Could you check a few things on this model? Use its own coordinates, in mm. A direction names the side the tool comes from. Round coordinates to 2 decimals unless told otherwise and drop trailing zeros. Loops run counter-clockwise (first coordinate to the right, second up) from the corner with the lowest first, then second, coordinate; pieces in that order, holes last. Notation, with made-up numbers: M 76,13 L 119,13 A16 ccw 119,25 Z; hole C 56.5,65.25 d6. An arc over 180 degrees is marked long. Return JSON: item names as keys, results as strings. Group by question number.
```python
from build123d import *

# Parameters (mm, degrees)
SKETCH1_W           = 25
SKETCH1_H           = 18
SKETCH1_R           = 3.5
BOSS_EXTRUDE1_DEPTH = 25
SKETCH2_W           = 20
SKETCH2_H           = 18
SKETCH2_R           = 3.96875
BOSS_EXTRUDE2_DEPTH = 4
FILLET2_R           = 3
FILLET4_R           = 3
SKETCH3_R           = 4.65
CUT_EXTRUDE1_DEPTH  = 22
SKETCH5_W           = 19
SKETCH5_H           = 12
CUT_EXTRUDE2_DEPTH  = 22
CHAMFER1_SIZE       = 1.25
CHAMFER1_SIZE2      = 4.665063509
CHAMFER2_SIZE       = 4.5
CHAMFER2_SIZE2      = 7.794228634
FILLET5_R           = 5.54
SKETCH7_W           = 3
SKETCH7_H           = 3
CUT_EXTRUDE3_DEPTH  = 6


with BuildPart() as part:
    # Sketch1 → Boss-Extrude1 (new body)
    with BuildSketch(Plane.XY):
        with Locations((12.5, 9)):
            Rectangle(SKETCH1_W, SKETCH1_H)
        with Locations((12.5, 9)):
            Circle(SKETCH1_R, mode=Mode.SUBTRACT)
    extrude(amount=BOSS_EXTRUDE1_DEPTH)

    # Sketch2 → Boss-Extrude2 (add)
    # profile 1 of 2: a face of its own
    with BuildSketch(Plane(origin=(0, 0, 0), x_dir=(-1, 0, 0), z_dir=(0, 0, -1))):
        with Locations((10, 9)):
            Rectangle(SKETCH2_W, SKETCH2_H)
        with Locations((10, 9)):
            Circle(SKETCH2_R, mode=Mode.SUBTRACT)
    # profile 2 of 2: a face of its own
    with BuildSketch(Plane(origin=(0, 0, 0), x_dir=(-1, 0, 0), z_dir=(0, 0, -1))):
        with Locations((-35, 9)):
            Rectangle(SKETCH2_W, SKETCH2_H)
        with Locations((-35, 9)):
            Circle(SKETCH2_R, mode=Mode.SUBTRACT)
    extrude(amount=-BOSS_EXTRUDE2_DEPTH)

    # Fillet2
    fillet2_edges = [part.edges().sort_by_distance(p)[0] for p in [
        (0, 9, 4),
        (-20, 0, 2),
        (-20, 18, 2),
        (45, 0, 2),
        (45, 18, 2),
        (25, 9, 4),
    ]]
    fillet(fillet2_edges, radius=FILLET2_R)

    # Fillet4
    fillet4_edges = [part.edges().sort_by_distance(p)[0] for p in [
        (12.5, 0, 25),
        (12.5, 18, 25),
        (0, 9, 25),
        (25, 9, 25),
    ]]
    fillet(fillet4_edges, radius=FILLET4_R)

    # Sketch3 → Cut-Extrude1 (cut)
    with BuildSketch(Plane(origin=(0, 0, 0), x_dir=(-1, 0, 0), z_dir=(0, 0, -1))):
        with Locations((-12.5, 9)):
            Circle(SKETCH3_R)
    extrude(amount=-CUT_EXTRUDE1_DEPTH, mode=Mode.SUBTRACT)

    # Sketch5 → Cut-Extrude2 (cut)
    with BuildSketch(Plane(origin=(0, 0, 0), x_dir=(-1, 0, 0), z_dir=(0, 0, -1))):
        with Locations((-12.5, 9)):
            Rectangle(SKETCH5_W, SKETCH5_H)
    extrude(amount=-CUT_EXTRUDE2_DEPTH, mode=Mode.SUBTRACT)

    # Chamfer1
    chamfer1_edges = [part.edges().sort_by_distance(p)[0] for p in [
        (12.5, 3, 22),
        (12.5, 15, 22),
    ]]
    chamfer1_side = [part.faces().sort_by_distance(p)[0] for p in [
        (12.5, 3.224722051, 22),
    ]]
    chamfer(chamfer1_edges, length=CHAMFER1_SIZE, length2=CHAMFER1_SIZE2, reference=chamfer1_side[0])

    # Chamfer2
    chamfer2_edges = [part.edges().sort_by_distance(p)[0] for p in [
        (22, 9, 22),
        (3, 9, 22),
    ]]
    chamfer2_side = [part.faces().sort_by_distance(p)[0] for p in [
        (21.787573542, 9, 22),
    ]]
    chamfer(chamfer2_edges, length=CHAMFER2_SIZE, length2=CHAMFER2_SIZE2, reference=chamfer2_side[0])

    # Fillet5
    # the kernel refuses this fillet: 5.54 mm, written as the material it adds along each edge
    with BuildSketch(Plane(origin=(13.422596023, 6.99868638, 32.258237225), x_dir=(-0.11302231218972587, 0.9741169476962979, -0.19576038710151827), z_dir=(-0.48705847384814693, -0.22604462437945333, -0.8436100229619524))) as fillet5_piece_1_section:
        with BuildLine():
            CenterArc((FILLET5_R * 0.877973148149, FILLET5_R), FILLET5_R, 187.435472226, 82.564527774)
            Line((-FILLET5_R * 0.113618085915, FILLET5_R * 0.870590477449), (0, 0))
            Line((0, 0), (FILLET5_R * 0.877973148149, 0))
        make_face()
    fillet5_piece_1 = extrude(amount=29.849737763, mode=Mode.PRIVATE)
    fillet5_piece_1 = split(fillet5_piece_1, bisect_by=Plane(origin=(6.414237593, 4.456810382, 22), z_dir=(0, 0, -1)), keep=Keep.TOP, mode=Mode.PRIVATE)
    fillet5_piece_1 = split(fillet5_piece_1, bisect_by=Plane(origin=(6.414237593, 0, 18.189685112), z_dir=(0, 1, 0)), keep=Keep.TOP, mode=Mode.PRIVATE)
    fillet5_piece_1 = split(fillet5_piece_1, bisect_by=Plane(origin=(0, 4.456810382, 18.189685112), z_dir=(1, 0, 0)), keep=Keep.TOP, mode=Mode.PRIVATE)
    add(fillet5_piece_1)
    with BuildSketch(Plane(origin=(11.577403977, 6.99868638, 32.258237225), x_dir=(-0.8733693623277119, -0.12606000911046675, -0.4704623588028643), z_dir=(0.48705847384814693, -0.2260446243794534, -0.8436100229619524))) as fillet5_piece_2_section:
        with BuildLine():
            CenterArc((FILLET5_R * 0.877973148149, FILLET5_R), FILLET5_R, 187.435472226, 82.564527774)
            Line((-FILLET5_R * 0.113618085915, FILLET5_R * 0.870590477449), (0, 0))
            Line((0, 0), (FILLET5_R * 0.877973148149, 0))
        make_face()
    fillet5_piece_2 = extrude(amount=29.849737763, mode=Mode.PRIVATE)
    fillet5_piece_2 = split(fillet5_piece_2, bisect_by=Plane(origin=(18.585762403, 4.456810384, 22), z_dir=(0, 0, -1)), keep=Keep.TOP, mode=Mode.PRIVATE)
    fillet5_piece_2 = split(fillet5_piece_2, bisect_by=Plane(origin=(18.585762403, 0, 18.189685124), z_dir=(0, 1, 0)), keep=Keep.TOP, mode=Mode.PRIVATE)
    fillet5_piece_2 = split(fillet5_piece_2, bisect_by=Plane(origin=(25, 4.456810384, 18.189685124), z_dir=(-1, 0, 0)), keep=Keep.TOP, mode=Mode.PRIVATE)
    add(fillet5_piece_2)
    with BuildSketch(Plane(origin=(11.577403977, 11.00131362, 32.258237225), x_dir=(0.11302231218972622, -0.9741169476962979, -0.19576038710151802), z_dir=(0.48705847384814693, 0.22604462437945327, -0.8436100229619524))) as fillet5_piece_3_section:
        with BuildLine():
            CenterArc((FILLET5_R * 0.877973148149, FILLET5_R), FILLET5_R, 187.435472226, 82.564527774)
            Line((-FILLET5_R * 0.113618085915, FILLET5_R * 0.870590477449), (0, 0))
            Line((0, 0), (FILLET5_R * 0.877973148149, 0))
        make_face()
    fillet5_piece_3 = extrude(amount=29.849737763, mode=Mode.PRIVATE)
    fillet5_piece_3 = split(fillet5_piece_3, bisect_by=Plane(origin=(18.585762407, 13.543189618, 22), z_dir=(0, 0, -1)), keep=Keep.TOP, mode=Mode.PRIVATE)
    fillet5_piece_3 = split(fillet5_piece_3, bisect_by=Plane(origin=(18.585762407, 18, 18.189685112), z_dir=(0, -1, 0)), keep=Keep.TOP, mode=Mode.PRIVATE)
    fillet5_piece_3 = split(fillet5_piece_3, bisect_by=Plane(origin=(25, 13.543189618, 18.189685112), z_dir=(-1, 0, 0)), keep=Keep.TOP, mode=Mode.PRIVATE)
    add(fillet5_piece_3)
    with BuildSketch(Plane(origin=(13.422596023, 11.00131362, 32.258237225), x_dir=(-0.11302231218972594, -0.9741169476962979, -0.1957603871015184), z_dir=(-0.4870584738481469, 0.22604462437945344, -0.8436100229619524))) as fillet5_piece_4_section:
        with BuildLine():
            CenterArc((FILLET5_R * 0.877973148149, -FILLET5_R), FILLET5_R, 90, 82.564527774)
            Line((-FILLET5_R * 0.113618085915, -FILLET5_R * 0.870590477449), (0, 0))
            Line((0, 0), (FILLET5_R * 0.877973148149, 0))
        make_face()
    fillet5_piece_4 = extrude(amount=29.849737763, mode=Mode.PRIVATE)
    fillet5_piece_4 = split(fillet5_piece_4, bisect_by=Plane(origin=(6.414237593, 13.543189618, 22), z_dir=(0, 0, -1)), keep=Keep.TOP, mode=Mode.PRIVATE)
    fillet5_piece_4 = split(fillet5_piece_4, bisect_by=Plane(origin=(6.414237593, 18, 18.189685112), z_dir=(0, -1, 0)), keep=Keep.TOP, mode=Mode.PRIVATE)
    fillet5_piece_4 = split(fillet5_piece_4, bisect_by=Plane(origin=(0, 13.543189618, 18.189685112), z_dir=(1, 0, 0)), keep=Keep.TOP, mode=Mode.PRIVATE)
    add(fillet5_piece_4)

    # Sketch7 → Cut-Extrude3 (cut)
    with BuildSketch(Plane(origin=(0, 0, 0), x_dir=(-1, 0, 0), z_dir=(0, 0, -1))):
        with Locations((-12.5, 1.5)):
            Rectangle(SKETCH7_W, SKETCH7_H)
    extrude(amount=-CUT_EXTRUDE3_DEPTH, mode=Mode.SUBTRACT)


solid = part.part
```
1. If we section it at A-A, the plane x = -10: Please give me the cut outline in (y, z).
2. If we section it at D-D, the plane y = 6.5: Give the number of separate pieces and of enclosed holes in the cut face, then the cut area to 3 significant figures.
3. We'd pull the mould along Y, two halves only. Please class faces 5 (the face through (7.168, 13.158, 18.745)), 6 (the face through (-19.1, 17.14, 2.03)), 7 (the face through (-20, 9, 2)): +Y half, -Y half, draft (parallel to the pull), parting line (faces both ways), or undercut.
4. I need wall thicknesses on probe 1 along Y at (x, z) = (10.5, 11.5); probe 2 along Y at (x, z) = (-10, 3.05); probe 3 along X at (y, z) = (7.5, 7.5). Which ranges of each line are inside material? Lowest first, please.
5. If we section it at B-B, the plane x = 32.5: Please give me the cut outline in (y, z), then the cut area to 3 significant figures.
6. I'm going to push flat-ended pins straight in: pin 1 Ø8 at (y, z) = (5.5, 15.5) entering from +X; pin 2 Ø4 at (x, y) = (22, 7.5) entering from -Z; pin 3 Ø10 at (y, z) = (9.5, 12.5) entering from -X; pin 4 Ø1.5 at (x, y) = (-4, 14) entering from +Z. Where does each tip first touch, or does it pass through?
7. On a 3-axis mill with a long thin cutter (end or side, diameter ignored), from which of +Z, -Z, +X, -X, +Y, -Y can I reach the whole of each face in a straight line? I mean faces 1 (the face through (12.53, 14.624, 18.74)), 2 (the face through (11, 1, 3)), 3 (the face through (39, 7, 4)), 4 (the face through (-0.9, 9.13, 4.86)). Say none if no direction works.
8. If we section it at C-C, the plane y = 17: Please give me the cut outline in (x, z), then the cut area to 3 significant figures.
Geometry results:
{
 "1": {"outline": "M 0,0 L 5.03,0 L 5.03,4 L 0,4 Z; M 12.97,0 L 18,0 L 18,4 L 12.97,4 Z"},
 "2": {"separate pieces": "4", "enclosed holes": "0", "area": "344 mm^2"},
 "3": {"face 5": "undercut", "face 6": "+Y half", "face 7": "draft"},
 "4": {"probe 1": "0 to 3, 15 to 18", "probe 2": "0 to 5.03, 12.97 to 18", "probe 3": "0 to 3, 22 to 25"},
 "5": {"outline": "M 0,0 L 5.92,0 L 5.92,4 L 0,4 Z; M 12.08,0 L 18,0 L 18,4 L 12.08,4 Z", "area": "47.3 mm^2"},
 "6": {"pin 1": "x = 25", "pin 2": "z = 0", "pin 3": "x = 0", "pin 4": "z = 4"},
 "7": {"face 1": "-Z", "face 2": "-Z, -Y", "face 3": "+Z, +X, +Y, -Y", "face 4": "+Z, -X, +Y, -Y"},
 "8": {"outline": "M -19.24,0 L 44.24,0 L 44.24,4 L 28,4 A3 cw 25,7 L 25,22 A3 ccw 24,24.24 L 1,24.24 A3 ccw 0,22 L 0,7 A3 cw -3,4 L -19.24,4 Z", "area": "762 mm^2"}
}
